Input: part model. Units: mm. Frame: model coordinates. Face numbers are marked on the shaded views. Coordinates: 2 decimals unless noted, no trailing zeros. Order: outer loops, then holes, each group sorted by start corner. A loop starts at its lowest first (then second) coordinate and runs counter-clockwise, first axis right, second up.
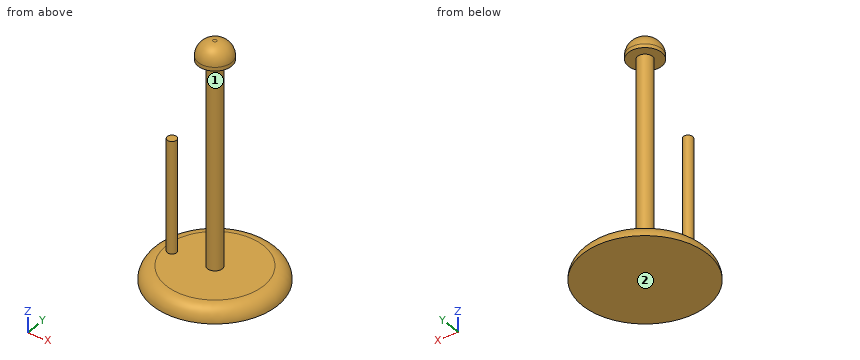
from build123d import *

# Parameters (mm, degrees)
F0_R     = 85.725
F1_DEPTH = 19.05
F2_R     = 19.04999
F3_R     = 10.16
F4_DEPTH = 279.4
F5_R     = 22.86
F6_DEPTH = 25.4
F7_R     = 20.32
F8_R     = 6.35
F9_DEPTH = 152.4


# Not quite as in the source:
# - a fillet or chamfer is up to 0.001 mm smaller than in the source, because OpenCascade refuses the exact size


with BuildPart() as f1:
    # F0 (on Top) → F1 (new body)
    with BuildSketch(Plane.XY):
        Circle(F0_R)
    extrude(amount=F1_DEPTH)

    # F2 (radius 19.05 in the source; OpenCascade refuses exactly that, so slightly less here)
    f2_edges = [f1.edges().sort_by_distance(p)[0] for p in [
        (-85.725, 0, 19.05),
    ]]
    fillet(f2_edges, radius=F2_R)

    # F3 (on face) → F4 (join)
    with BuildSketch(Plane.XY.offset(19.05)):
        Circle(F3_R)
    extrude(amount=F4_DEPTH)

    # F5 (on face) → F6 (join)
    with BuildSketch(Plane.XY.offset(298.45)):
        Circle(F5_R)
    extrude(amount=F6_DEPTH)

    # F7
    f7_edges = [f1.edges().sort_by_distance(p)[0] for p in [
        (-22.86, 0, 323.85),
    ]]
    fillet(f7_edges, radius=F7_R)

    # F8 (on face) → F9 (join)
    with BuildSketch(Plane.XY.offset(19.05)):
        with Locations((-55.5577278137, -4.9048527144)):
            Circle(F8_R)
    extrude(amount=F9_DEPTH)


solid = f1.part
Item 1: Cut plane A-A on z = 134. Return loops of the section in (x, y), then the cut area to 3 significant figures.
Response values:
outline: circle Ø12.7 at (-55.56, -4.9); circle Ø20.32 at (0, 0)
area: 451 mm2
Item 2: Ray query, probe 1 along Z at (x, y) = (-22, -59); probe 2 along X at (y, z) = (-5, 28.5); probe 3 along Z at (x, y) = (37.5, -71). Return the intervals inside material, ascending.
Response values:
probe 1: z = 0 to 19.05
probe 2: x = -61.91 to -49.21, -8.84 to 8.84
probe 3: z = 0 to 13.32
Item 3: Draft query along Z for the marked faces 1 and 2. Return one class per face: pulls with the +Z half, pulls with the -Z half, needs draft (parallel to the pull), parting line crosses it, or undercut.
Response values:
face 1: undercut
face 2: pulls with the -Z half
Item 4: Pin query (flat end, axial travel): pin 1 Ø1.5 at (x, z) = (-3.5, 265.5) entering from +Y; pin 2 Ø6 at (x, y) = (49.5, -59.5) entering from +Z; pin 3 Ø14 at (x, y) = (-54.5, -4.5) entering from +Z. Return the tip coordinate at first contact, or that it passes through.
Response values:
pin 1: stops at y = 9.78
pin 2: stops at z = 17.41
pin 3: stops at z = 171.45
Item 5: Cut plane B-B on z = 271. Return loops of the section in (x, y), then the cut area to 3 significant figures.
Response values:
outline: circle Ø20.32 at (0, 0)
area: 324 mm2
